Geometry check sheet. Reference: the model listing, model coordinates, mm. Face numbers are marked on the shaded views. A direction names the side the tool comes from. Give positions to 0.01 mm unless a question says otherwise; leave off trailing zeros.
from build123d import *

# Parameters (mm, degrees)
F0_R     = 13.57391
F1_DEPTH = 17
F3_DEPTH = 1.5
F5_DEPTH = 34
F6_R     = 1
F7_R     = 15.57391
F7_R_2   = 13.57391
F8_DEPTH = 1.5
F9_SIZE2 = 0.99999
F9_SIZE  = 1.99999
F10_R    = 1


# Not quite as in the source:
# - a fillet or chamfer is up to 0.001 mm smaller than in the source, because OpenCascade refuses the exact size


with BuildPart() as f1:
    # F0 (on Top) → F1 (new body, symmetric)
    with BuildSketch(Plane.XY):
        Circle(F0_R)
    extrude(amount=F1_DEPTH, both=True)

    # F2 (on Top) → F3 (join, symmetric)
    with BuildSketch(Plane.XY):
        with BuildLine():
            Line((-8.8722387473, 10.27299432), (-13.094084175, 11.721231689))
            ThreePointArc((-13.094084175, 11.721231689), (-13.7398361081, 10.9571536638), (-14.3410637787, 10.1575687241))
            Line((-14.3410637787, 10.1575687241), (-11.9896877566, 6.3638369077))
            ThreePointArc((-11.9896877566, 6.3638369077), (-10.6125101782, 8.4631944563), (-8.8722387473, 10.27299432))
        make_face()
        with BuildLine():
            ThreePointArc((1, 17.5454356654), (0, 17.57391), (-1, 17.5454356654))
            Line((-1, 17.5454356654), (-2.5, 13.3417027657))
            ThreePointArc((-2.5, 13.3417027657), (0, 13.57391), (2.5, 13.3417027657))
            Line((2.5, 13.3417027657), (1, 17.5454356654))
        make_face()
        with BuildLine():
            Line((11.9896877566, 6.3638369077), (14.3410637787, 10.1575687241))
            ThreePointArc((14.3410637787, 10.1575687241), (13.7398361081, 10.9571536638), (13.094084175, 11.721231689))
            Line((13.094084175, 11.721231689), (8.8722387473, 10.27299432))
            ThreePointArc((8.8722387473, 10.27299432), (10.6125101782, 8.4631944563), (11.9896877566, 6.3638369077))
        make_face()
        with BuildLine():
            Line((12.4508960874, -5.4061279404), (16.8830140276, -4.8791546431))
            ThreePointArc((16.8830140276, -4.8791546431), (17.1332953852, -3.9105628665), (17.3280558955, -2.9292988187))
            Line((17.3280558955, -2.9292988187), (13.5635007572, -0.5314883795))
            ThreePointArc((13.5635007572, -0.5314883795), (13.2335837364, -3.0204791306), (12.4508960874, -5.4061279404))
        make_face()
        with BuildLine():
            Line((3.5363257124, -13.1051681845), (6.711710363, -16.2417750474))
            ThreePointArc((6.711710363, -16.2417750474), (7.6250337817, -15.8335457973), (8.5136480988, -15.3740075692))
            Line((8.5136480988, -15.3740075692), (8.0411700519, -10.9357494889))
            ThreePointArc((8.0411700519, -10.9357494889), (5.8894988252, -12.2296703257), (3.5363257124, -13.1051681845))
        make_face()
        with BuildLine():
            Line((-8.0411700519, -10.9357494889), (-8.5136480988, -15.3740075692))
            ThreePointArc((-8.5136480988, -15.3740075692), (-7.6250337817, -15.8335457973), (-6.711710363, -16.2417750474))
            Line((-6.711710363, -16.2417750474), (-3.5363257124, -13.1051681845))
            ThreePointArc((-3.5363257124, -13.1051681845), (-5.8894988252, -12.2296703257), (-8.0411700519, -10.9357494889))
        make_face()
        with BuildLine():
            Line((-13.5635007572, -0.5314883795), (-17.3280558955, -2.9292988187))
            ThreePointArc((-17.3280558955, -2.9292988187), (-17.1332953852, -3.9105628665), (-16.8830140276, -4.8791546431))
            Line((-16.8830140276, -4.8791546431), (-12.4508960874, -5.4061279404))
            ThreePointArc((-12.4508960874, -5.4061279404), (-13.2335837364, -3.0204791306), (-13.5635007572, -0.5314883795))
        make_face()
    extrude(amount=F3_DEPTH, both=True)

    # F4 (on face) → F5 (cut)
    with BuildSketch(Plane.XY.offset(17)):
        with BuildLine():
            ThreePointArc((-3.0007085232, 1.5847516846), (-2.6531275445, 2.1157986141), (-2.2127391143, 2.5728340707))
            Line((-2.2127391143, 2.5728340707), (-6.6382173429, 7.718502212))
            ThreePointArc((-6.6382173429, 7.718502212), (-7.9593826336, 6.3473958423), (-9.0021255696, 4.7542550537))
            Line((-9.0021255696, 4.7542550537), (-3.0007085232, 1.5847516846))
        make_face()
        with BuildLine():
            ThreePointArc((-0.6319024037, 3.334124907), (-0.3173418417, 3.3786067688), (0, 3.3934775))
            Line((0, 3.3934775), (0, 6.786955))
            Line((0, 6.786955), (0, 10.1804325))
            ThreePointArc((0, 10.1804325), (-0.9520255252, 10.1358203065), (-1.895707211, 10.0023747209))
            Line((-1.895707211, 10.0023747209), (-0.6319024037, 3.334124907))
        make_face()
        with BuildLine():
            Line((0, 6.786955), (0, 3.3934775))
            ThreePointArc((0, 3.3934775), (0.3173418417, 3.3786067688), (0.6319024037, 3.334124907))
            Line((0.6319024037, 3.334124907), (1.895707211, 10.0023747209))
            ThreePointArc((1.895707211, 10.0023747209), (0.9520255252, 10.1358203065), (0, 10.1804325))
            Line((0, 10.1804325), (0, 6.786955))
        make_face()
        with BuildLine():
            ThreePointArc((2.2127391143, 2.5728340707), (2.6531275445, 2.1157986141), (3.0007085232, 1.5847516846))
            Line((3.0007085232, 1.5847516846), (9.0021255696, 4.7542550537))
            ThreePointArc((9.0021255696, 4.7542550537), (7.9593826336, 6.3473958423), (6.6382173429, 7.718502212))
            Line((6.6382173429, 7.718502212), (2.2127391143, 2.5728340707))
        make_face()
        with BuildLine():
            ThreePointArc((3.3911429475, -0.1258532971), (3.3083959341, -0.7551197827), (3.1099199215, -1.3579718793))
            Line((3.1099199215, -1.3579718793), (9.3297597644, -4.073915638))
            ThreePointArc((9.3297597644, -4.073915638), (9.9251878023, -2.265359348), (10.1734288426, -0.3775598913))
            Line((10.1734288426, -0.3775598913), (3.3911429475, -0.1258532971))
        make_face()
        with BuildLine():
            ThreePointArc((2.0159469746, -2.7297705652), (1.4723747063, -3.0574175814), (0.8772981881, -3.2781149205))
            Line((0.8772981881, -3.2781149205), (2.6318945642, -9.8343447616))
            ThreePointArc((2.6318945642, -9.8343447616), (4.4171241189, -9.1722527443), (6.0478409237, -8.1893116956))
            Line((6.0478409237, -8.1893116956), (2.0159469746, -2.7297705652))
        make_face()
        with BuildLine():
            ThreePointArc((-0.8772981881, -3.2781149205), (-1.4723747063, -3.0574175814), (-2.0159469746, -2.7297705652))
            Line((-2.0159469746, -2.7297705652), (-6.0478409237, -8.1893116956))
            ThreePointArc((-6.0478409237, -8.1893116956), (-4.4171241189, -9.1722527443), (-2.6318945642, -9.8343447616))
            Line((-2.6318945642, -9.8343447616), (-0.8772981881, -3.2781149205))
        make_face()
        with BuildLine():
            ThreePointArc((-3.1099199215, -1.3579718793), (-3.3083959341, -0.7551197827), (-3.3911429475, -0.1258532971))
            Line((-3.3911429475, -0.1258532971), (-10.1734288426, -0.3775598913))
            ThreePointArc((-10.1734288426, -0.3775598913), (-9.9251878023, -2.265359348), (-9.3297597644, -4.073915638))
            Line((-9.3297597644, -4.073915638), (-3.1099199215, -1.3579718793))
        make_face()
        Polygon((-1.2990381057, 0.68605558), (0, 0), (-0.8620256343, 1.002309268), (-1.2990381057, 0.75), align=None)
        Polygon((-0.8620256343, 1.002309268), (0, 0), (-0.2562490973, 1.3520545147), align=None)
        Polygon((-0.2562490973, 1.3520545147), (0, 0), (0, 1.5), align=None)
        Polygon((0, 1.5), (0, 0), (0.2562490973, 1.3520545147), align=None)
        Polygon((0.2562490973, 1.3520545147), (0, 0), (0.8620256343, 1.002309268), align=None)
        Polygon((0.8620256343, 1.002309268), (0, 0), (1.2990381057, 0.68605558), (1.2990381057, 0.75), align=None)
        Polygon((1.2990381057, 0.68605558), (0, 0), (1.2990381057, -0.0482103619), align=None)
        Polygon((1.2990381057, -0.0482103619), (0, 0), (1.2990381057, -0.5672355759), align=None)
        Polygon((1.2990381057, -0.5672355759), (0, 0), (0.7766231283, -1.0516164278), (1.2990381057, -0.75), align=None)
        Polygon((0.7766231283, -1.0516164278), (0, 0), (0.3477089236, -1.2992501593), align=None)
        Polygon((0.3477089236, -1.2992501593), (0, 0), (-0.3477089236, -1.2992501593), (0, -1.5), align=None)
        Polygon((-0.3477089236, -1.2992501593), (0, 0), (-0.7766231283, -1.0516164278), align=None)
        Polygon((-0.7766231283, -1.0516164278), (0, 0), (-1.2990381057, -0.5672355759), (-1.2990381057, -0.75), align=None)
        Polygon((-1.2990381057, -0.5672355759), (0, 0), (-1.2990381057, -0.0482103619), align=None)
        Polygon((-1.2990381057, -0.0482103619), (0, 0), (-1.2990381057, 0.68605558), align=None)
    extrude(amount=-F5_DEPTH, mode=Mode.SUBTRACT)

    # F6
    f6_edges = [f1.edges().sort_by_distance(p)[0] for p in [
        (-6.047841, -8.189312, 0),
        (-2.631895, -9.834345, 0),
        (2.631895, -9.834345, 0),
        (6.047841, -8.189312, 0),
        (9.32976, -4.073916, 0),
        (-9.32976, -4.073916, 0),
        (-10.173429, -0.37756, 0),
        (-9.002126, 4.754255, 0),
        (-6.638217, 7.718502, 0),
        (6.638217, 7.718502, 0),
        (-1.895707, 10.002375, 0),
        (1.895707, 10.002375, 0),
        (9.002126, 4.754255, 0),
        (10.173429, -0.37756, 0),
    ]]
    fillet(f6_edges, radius=F6_R)

    # F7 (on face) → F8 (join)
    with BuildSketch(Plane(origin=(0, 0, -17), x_dir=(1, 0, 0), z_dir=(0, 0, -1))):
        Circle(F7_R)
        Circle(F7_R_2, mode=Mode.SUBTRACT)
    extrude(amount=-F8_DEPTH)

    # F9 (size 2 and 1 in the source; OpenCascade refuses exactly that, so slightly less here)
    f9_edges = [f1.edges().sort_by_distance(p)[0] for p in [
        (-15.57391, 0, -15.5),
    ]]
    f9_side = f1.faces().sort_by_distance((-15.133413, 0, -15.5))[0]
    chamfer(f9_edges, length=F9_SIZE, length2=F9_SIZE2, reference=f9_side)

    # F10
    f10_edges = [f1.edges().sort_by_distance(p)[0] for p in [
        (14.341064, 10.157569, 0),
        (13.094084, 11.721232, 0),
        (1, 17.545436, 0),
        (-1, 17.545436, 0),
        (-13.094084, 11.721232, 0),
        (-14.341064, 10.157569, 0),
        (-17.328056, -2.929299, 0),
        (-16.883014, -4.879155, 0),
        (-8.513648, -15.374008, 0),
        (-6.71171, -16.241775, 0),
        (6.71171, -16.241775, 0),
        (8.513648, -15.374008, 0),
        (16.883014, -4.879155, 0),
        (17.328056, -2.929299, 0),
    ]]
    fillet(f10_edges, radius=F10_R)


solid = f1.part
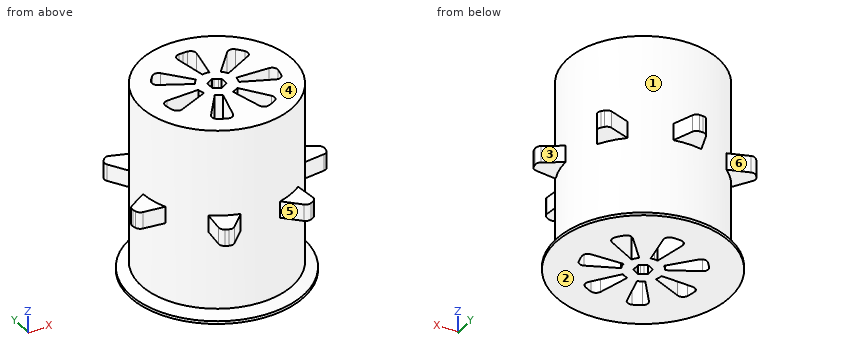
Item 1: Draft check along Y on the marked faces 3, 4, 5 and 6. Enter one of: released by +Y, released by -Y, zero draft, split by the parting line, or undercut.
Reported:
face 3: undercut
face 4: zero draft
face 5: released by -Y
face 6: released by +Y
Item 2: Scan lines: L1, parallel to Y at x = 7, z = -6.5; L2, parallel to Y at x = 5, z = 2; L3, parallel to X at y = 0, z = -15. Record each from-to range of solid material in increasing order.
Reported:
L1: y = -11.63 to -3.06, -0.26 to 3.7, 7.22 to 11.63
L2: y = -12.62 to -8.87, -6.77 to -2.18, -0.19 to 2.64, 5.81 to 12.62
L3: x = -13.57 to -1.3, 1.3 to 13.57
Item 3: Gauge pin test, flat ends, axial feed: pin 1 (2.5 mm diameter, centred on x = -15.5, y = -3.5, fed in from -Z); pin 2 (1.3 mm diameter, centred on x = -0.5, y = 16.5, fed in from +Z); pin 3 (1 mm diameter, centred on y = -5.5, z = 5, fed in from +X); pin 4 (4 mm diameter, centred on x = 12.5, z = 13, fed in from -Y). Record the tip position at first contact, or that the pin passes through.
Reported:
pin 1: stops at z = -17
pin 2: stops at z = 1.5
pin 3: stops at x = 12.62
pin 4: stops at y = -8.6
Item 4: Sectioned sample at A-A (z = 3). Give the number of separate pieces and of enclosed holes in the cut face, and give its area (3 significant figures).
Reported:
separate pieces: 1
enclosed holes: 8
area: 456 mm2
Item 5: Set-up check for the marked faces 1 and 2: record each of +Z, -Z, +X, -X, +Y, -Y from which the full face is reachable in a straight line by a thin tool's end or side.
Reported:
face 1: none
face 2: -Z, +X, -X, +Y, -Y
